Could you check a few things on this drawing? It's one solid part, dimensions in mm from its lowest x, y, z. A direction names the side the tool comes from. Round coordinates to 2 decimals unless told otherwise and drop trailing zeros. Loops run counter-clockwise (first coordinate to the right, second up) from the corner with the lowest first, then second, coordinate; pieces in that order, holes last. Notation, with made-up numbers: M 88,31 L 121,31 A14 cw 121,46 Z; hole C 37,47 d4. An arc over 180 degrees is marked long. Write each question's results on one line, items separated by ' | '. Start each with the question number.
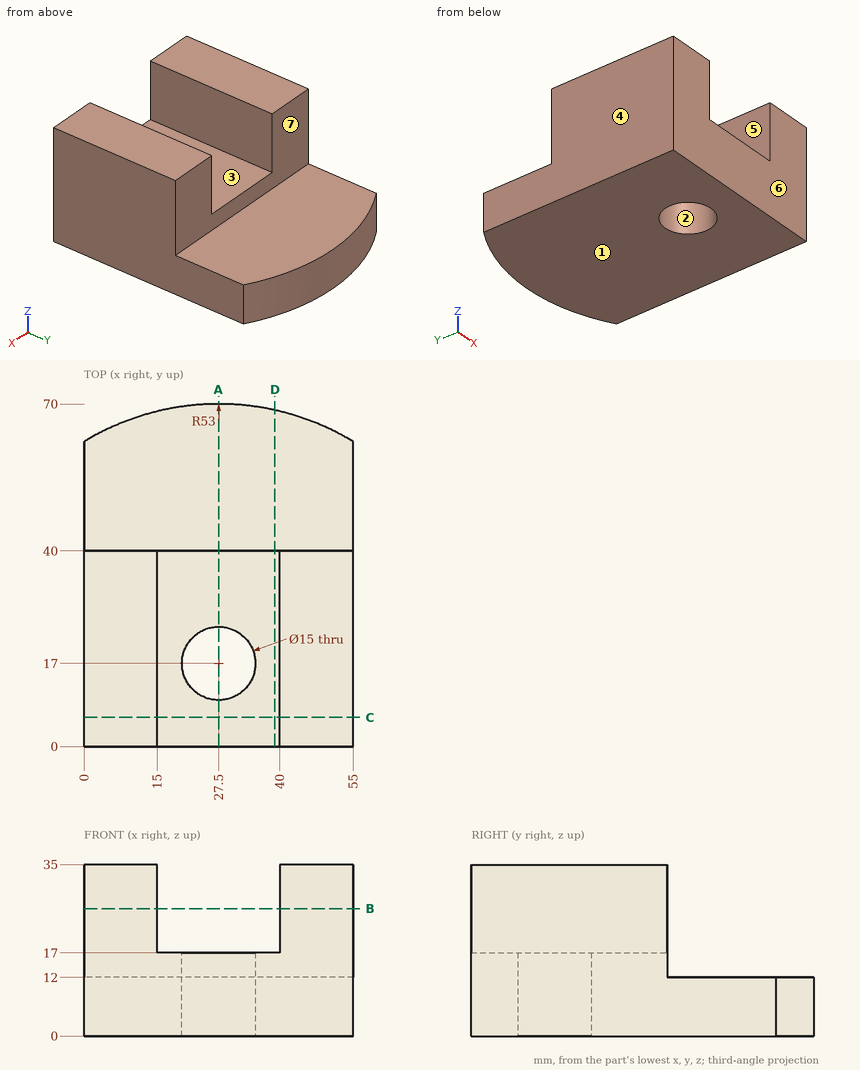
1. I want a section at C-C on y = 6. List the corners of the cut face in (x, z) for me.
2. For pin 1 (8 mm diameter, centred on y = 46.5, z = 20.5, fed in from -X); pin 2 (5 mm diameter, centred on x = 31.5, y = 50.5, fed in from +Z); pin 3 (12 mm diameter, centred on x = 45.5, z = 8.5, fed in from +Y); pin 4 (12 mm diameter, centred on x = 25.5, y = 40, fed in from +Z), each with a flat end and sliding along its axis, tell me the tip position at first contact or that it passes through.
3. I want a section at A-A on x = 27.5. List the corners of the cut face in (y, z) for me.
4. I want a section at D-D on x = 39. List the corners of the cut face in (y, z) for me.
5. Which directions (+Z, -Z, +X, -X, +Y, -Y) give clear straight access to the entire face, cutting with the end or side of a thin tool? Please do the marked faces 5, 6 and 7.
6. I need wall thicknesses on line 1 along X through (y, z) = (28, 22); line 2 along Y through (x, z) = (27.5, 7); line 3 along Y through (x, z) = (3.5, 22). Which ranges of each line are inside material? Lowest first, please.
7. If we mould it in two halves opening along X, with no side actions, what happens to the marked faces 1, 2, 3 and 4? For each: released by +X, released by -X, zero draft, split by the parting line, or undercut.
8. I want a section at B-B on z = 26. List the corners of the cut face in (x, y) for me.
Outcome:
1) outline: M 0,0 L 55,0 L 55,35 L 40,35 L 40,17 L 15,17 L 15,35 L 0,35 Z
2) pin 1: through | pin 2: z = 12 | pin 3: y = 68.62 | pin 4: z = 17
3) outline: M 0,0 L 9.5,0 L 9.5,17 L 0,17 Z; M 24.5,0 L 70,0 L 70,12 L 40,12 L 40,17 L 24.5,17 Z
4) outline: M 0,0 L 68.74,0 L 68.74,12 L 40,12 L 40,17 L 0,17 Z
5) face 5: +Z, +Y, -Y | face 6: +Z, -Z, +X, -X, -Y | face 7: +Z, +X, -X, +Y
6) line 1: 0 to 15, 40 to 55 | line 2: 0 to 9.5, 24.5 to 70 | line 3: 0 to 40
7) face 1: zero draft | face 2: undercut | face 3: undercut | face 4: released by -X
8) outline: M 0,0 L 15,0 L 15,40 L 0,40 Z; M 40,0 L 55,0 L 55,40 L 40,40 Z
